For this review, use the dimensioned drawing (mm, ordinates from the lowest corner) and the shaded views. A direction names the side the tool comes from. Coordinates: 2 decimals unless noted, no trailing zeros. Write each loop counter-clockwise with the first axis right and the second up, starting at its lowest first coordinate (ties: lowest second). Pieces come first, ordered by that corner, then holes. Notation, with made-up numbers: M -30,-35.5 L 8,-35.5 A28 ccw 8,2.5 Z; hole C -20.75,77 d10. An arc over 180 degrees is marked long. Return JSON: item names as keys, results as strings.
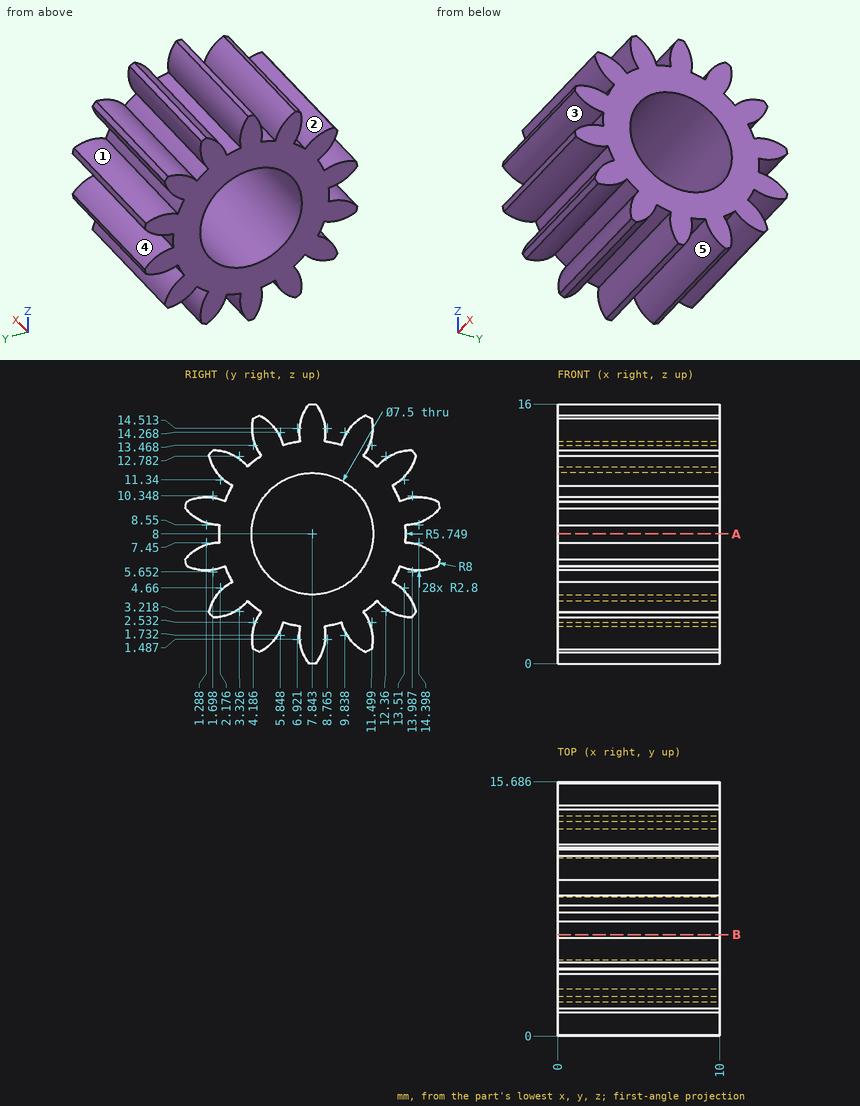
1. Wall thickness on L1, parallel to Y at x = 3.5, z = 8; L2, parallel to Z at x = 5.75, y = 13.5 (1 decimal); L3, parallel to Y at x = 2.5, z = 12.25 (1 decimal): over which ranges is each line inside the solid? List them lowest first. Write a range as from..to.
Checks:
{"L1": "2.09..4.09, 11.59..13.59", "L2": "2.9..4.5, 5.9..10.1, 11.5..13.1", "L3": "1.7..3.8, 4..11.7, 11.9..14"}
2. We need section A-A (z = 8). State the section outline as (x, y) points.
Checks:
{"outline": "M 0,2.09 L 10,2.09 L 10,4.09 L 0,4.09 Z; M 0,11.59 L 10,11.59 L 10,13.59 L 0,13.59 Z"}
3. For the marked faces 1, 2, 3, 4 and 5, list the 3-axis set-ups (+Z, -Z, +X, -X, +Y, -Y) from which the entire face can be reached by the end or side of a thin tool; tool diameter is ignored.
Checks:
{"face 1": "+X, -X", "face 2": "+Z, +X, -X", "face 3": "+X, -X, -Y", "face 4": "+X, -X, +Y", "face 5": "-Z, +X, -X"}
4. We need section B-B (y = 6.25). State the section outline as (x, z) points (1 decimal).
Checks:
{"outline": "M 0,2.5 L 10,2.5 L 10,4.6 L 0,4.6 Z; M 0,11.4 L 10,11.4 L 10,13.5 L 0,13.5 Z"}
5. Clearance check with flat-ended pins moving along their axes: pin 1 Ø6 at (x, y) = (9, 13.5) entering from +Z (1 decimal); pin 2 Ø2 at (x, y) = (9, 2.5) entering from -Z. State where each tip first meets the part, or that it passes through.
Checks:
{"pin 1": "z = 15.3", "pin 2": "z = 2.85"}
